Here's how the part is built. I have some questions about the finished solid (model axes, mm). Face numbers are marked on the shaded views. Round coordinates to 2 decimals unless told otherwise and drop trailing zeros. Write each loop counter-clockwise with the first axis right and the second up, starting at its lowest first coordinate (ties: lowest second). Pieces come first, ordered by that corner, then holes. Notation, with made-up numbers: (-8, -22.75) - (1, -22.75) arc R18 ccw to (1, -11.75) - close; hole circle Ø1 at (62, -35). An arc over 180 degrees is marked (long way). Write item = value, one per line. Start each with the question number.
Item 1: If we section it at D-D (x = 34.5): Please give me the cut outline in (y, z).
Item 2: If I drill on line 1 along Z through (x, y) = (-41, 0.85); line 2 along Z through (x, y) = (-0.5, 0.7); line 3 along X through (y, z) = (2.6, -40.5), over which ranges is the centre line in solid material (lowest first)? Write a range as [from, to].
Item 3: If we section it at A-A (x = -42.5): Please give me the cut outline in (y, z).
Item 4: If we section it at B-B (y = 1.95): Please give me the cut outline in (x, z), and give its area (3 significant figures).
Item 5: Thinking about a two-plate mould opening in Y: for the marked faces 1 and 2, which applies, pulls with the +Y half, pulls with the -Y half, needs draft (parallel to the pull), parting line crosses it, or undercut?
Item 6: If we section it at C-C (z = 15): Please give me the cut outline in (x, y).
Item 7: For P1, Ø1.5, axis at y = 2, z = -61, coming from the +X side; P2, Ø1, axis at x = 7.5, y = 0.5, coming from the -Z side, each with a flat end and sliding along its axis, tell me the tip position at first contact or that it passes through.
```python
from build123d import *

# Parameters (mm, degrees)
SKETCH1_R           = 3.2
BOSS_EXTRUDE1_DEPTH = 3


with BuildPart() as part:
    # Sketch1 → Boss-Extrude1 (new body)
    with BuildSketch(Plane(origin=(0, 0, 0), x_dir=(1, 0, 0), z_dir=(0, 1, 0))):
        with BuildLine():
            Line((-46.074522422, 10.719183363), (-37.235687657, 19.558018127))
            Line((-37.235687657, 19.558018127), (-74.493699398, 56.816029868))
            Line((-74.493699398, 56.816029868), (-83.332534163, 65.654864633))
            ThreePointArc((-83.332534163, 65.654864633), (-83.332534163, 83.332534163), (-65.654864633, 83.332534163))
            Line((-65.654864633, 83.332534163), (-56.816029868, 74.493699398))
            Line((-56.816029868, 74.493699398), (-19.558018127, 37.235687657))
            Line((-19.558018127, 37.235687657), (-10.719183363, 46.074522422))
            ThreePointArc((-10.719183363, 46.074522422), (0, 50.514553548), (10.719183363, 46.074522422))
            Line((10.719183363, 46.074522422), (46.074522422, 10.719183363))
            ThreePointArc((46.074522422, 10.719183363), (50.514553548, 0), (46.074522422, -10.719183363))
            Line((46.074522422, -10.719183363), (37.235687657, -19.558018127))
            Line((37.235687657, -19.558018127), (74.493699398, -56.816029868))
            Line((74.493699398, -56.816029868), (83.332534163, -65.654864633))
            ThreePointArc((83.332534163, -65.654864633), (83.332534163, -83.332534163), (65.654864633, -83.332534163))
            Line((65.654864633, -83.332534163), (56.816029868, -74.493699398))
            Line((56.816029868, -74.493699398), (19.558018127, -37.235687657))
            Line((19.558018127, -37.235687657), (10.719183363, -46.074522422))
            ThreePointArc((10.719183363, -46.074522422), (0, -50.514553548), (-10.719183363, -46.074522422))
            Line((-10.719183363, -46.074522422), (-46.074522422, -10.719183363))
            ThreePointArc((-46.074522422, -10.719183363), (-50.514553548, 0), (-46.074522422, 10.719183363))
        make_face()
        with Locations((56.674608512, -56.674608512)):
            Circle(SKETCH1_R, mode=Mode.SUBTRACT)
        with Locations((-56.674608512, 56.674608512)):
            Circle(SKETCH1_R, mode=Mode.SUBTRACT)
    extrude(amount=BOSS_EXTRUDE1_DEPTH)


solid = part.part
```
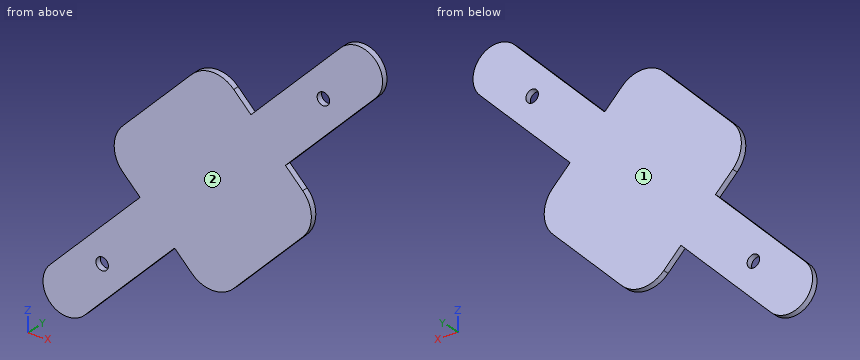
Reply:
q1.outline = (0, -22.29) - (3, -22.29) - (3, 52.18) - (0, 52.18) - close
q2.line_1 = [-58.68, -23.32], [-15.79, 15.79]
q2.line_2 = [-50.51, 50.51]
q2.line_3 = [-58.18, -22.82], [-16.29, 16.29]
q3.outline = (0, -60.18) - (3, -60.18) - (3, -24.82) - (0, -24.82) - close; (0, -14.29) - (3, -14.29) - (3, 14.29) - (0, 14.29) - close
q4.outline = (-83.33, -65.65) arc R12.5 ccw to (-65.65, -83.33) - (-19.56, -37.24) - (-10.72, -46.07) arc R15.16 ccw to (10.72, -46.07) - (46.07, -10.72) arc R15.16 ccw to (46.07, 10.72) - (37.24, 19.56) - (83.33, 65.65) arc R12.5 ccw to (65.65, 83.33) - (19.56, 37.24) - (10.72, 46.07) arc R15.16 ccw to (-10.72, 46.07) - (-46.07, 10.72) arc R15.16 ccw to (-46.07, -10.72) - (-37.24, -19.56) - close; hole circle Ø6.4 at (-56.67, -56.67); hole circle Ø6.4 at (56.67, 56.67)
q4.area = 9,940 mm2
q5.face_1 = pulls with the +Y half
q5.face_2 = pulls with the -Y half
q6.outline = (-41.79, 0) - (41.79, 0) - (41.79, 3) - (-41.79, 3) - close
q7.P1 = -42.57
q7.P2 = -48.8
